Part model, mm, in its own coordinate system. A direction names the side the tool comes from. Round coordinates to 2 decimals unless told otherwise and drop trailing zeros. Write each loop counter-clockwise with the first axis right and the second up, starting at its lowest first coordinate (ties: lowest second). Pieces come first, ordered by that corner, then holes.
```python
from build123d import *

# Parameters (mm, degrees)
SKETCH1_W                = 57
SKETCH1_H                = 57
EXTRUDE1_DEPTH           = 76
F_5_0_5_DIAMETER_HOLE1_D = 5
SKETCH6_R                = 4
SKETCH6_R_2              = 2.5
EXTRUDE4_DEPTH           = 71
FILLET1_R                = 5
SKETCH7_R                = 3
EXTRUDE5_DEPTH           = 101
SKETCH8_R                = 19.05
EXTRUDE6_DEPTH           = 3
FILLET2_R                = 1
SKETCH9_R                = 5.5
BOSS_EXTRUDE1_DEPTH      = 388
CHAMFER1_SIZE            = 0.5
SKETCH10_R               = 4
BOSS_EXTRUDE2_DEPTH      = 10
CHAMFER2_SIZE            = 0.5


with BuildPart() as part:
    # Sketch1 → Extrude1 (new body)
    with BuildSketch(Plane(origin=(0, 0, 0), x_dir=(1, 0, 0), z_dir=(0, 1, 0))):
        Rectangle(SKETCH1_W, SKETCH1_H)
    extrude(amount=EXTRUDE1_DEPTH)

    # Ø5.0 (5) Diameter Hole1 (through all)
    with Locations(Plane.XZ):
        with Locations((-23.5, 23.5), (23.5, 23.5), (23.5, -23.5), (-23.5, -23.5)):
            Hole(F_5_0_5_DIAMETER_HOLE1_D / 2)

    # Sketch6 → Extrude4 (cut)
    # profile 1 of 12: a face of its own
    with BuildSketch(Plane(origin=(0, 76, 0), x_dir=(1, 0, 0), z_dir=(0, 1, 0))):
        Polygon((-28.5, 28.5), (-19.5, 28.5), (-19.5, 32.511741208), (-33.908905561, 32.511741208), (-33.908905561, 19.5), (-28.5, 19.5), align=None)
    # profile 2 of 12: a face of its own
    with BuildSketch(Plane(origin=(0, 76, 0), x_dir=(1, 0, 0), z_dir=(0, 1, 0))):
        with BuildLine():
            ThreePointArc((-23.5, 19.5), (-26.328427125, 26.328427125), (-19.5, 23.5))
            Line((-19.5, 23.5), (-19.5, 28.5))
            Line((-19.5, 28.5), (-28.5, 28.5))
            Line((-28.5, 28.5), (-28.5, 19.5))
            Line((-28.5, 19.5), (-23.5, 19.5))
        make_face()
    # profile 3 of 12: a face of its own
    with BuildSketch(Plane(origin=(0, 76, 0), x_dir=(1, 0, 0), z_dir=(0, 1, 0))):
        with Locations((-23.5, 23.5)):
            Circle(SKETCH6_R)
        with Locations(Location((-23.5, 23.5, 0), (0, 0, 90))):
            Circle(SKETCH6_R_2, mode=Mode.SUBTRACT)
    # profile 4 of 12: a face of its own
    with BuildSketch(Plane(origin=(0, 76, 0), x_dir=(1, 0, 0), z_dir=(0, 1, 0))):
        Polygon((19.5, 36.471560472), (19.5, 28.5), (28.5, 28.5), (28.5, 19.5), (41.168352552, 19.5), (41.168352552, 36.471560472), align=None)
    # profile 5 of 12: a face of its own
    with BuildSketch(Plane(origin=(0, 76, 0), x_dir=(1, 0, 0), z_dir=(0, 1, 0))):
        with BuildLine():
            Line((28.5, 28.5), (19.5, 28.5))
            Line((19.5, 28.5), (19.5, 23.5))
            ThreePointArc((19.5, 23.5), (23.5, 27.5), (27.5, 23.5))
            ThreePointArc((27.5, 23.5), (26.328427125, 20.671572875), (23.5, 19.5))
            Line((23.5, 19.5), (28.5, 19.5))
            Line((28.5, 19.5), (28.5, 28.5))
        make_face()
    # profile 6 of 12: a face of its own
    with BuildSketch(Plane(origin=(0, 76, 0), x_dir=(1, 0, 0), z_dir=(0, 1, 0))):
        with Locations((23.5, 23.5)):
            Circle(SKETCH6_R)
        with Locations(Location((23.5, 23.5, 0), (0, 0, 90))):
            Circle(SKETCH6_R_2, mode=Mode.SUBTRACT)
    # profile 7 of 12: a face of its own
    with BuildSketch(Plane(origin=(0, 76, 0), x_dir=(1, 0, 0), z_dir=(0, 1, 0))):
        with Locations((23.5, -23.5)):
            Circle(SKETCH6_R)
        with Locations(Location((23.5, -23.5, 0), (0, 0, 90))):
            Circle(SKETCH6_R_2, mode=Mode.SUBTRACT)
    # profile 8 of 12: a face of its own
    with BuildSketch(Plane(origin=(0, 76, 0), x_dir=(1, 0, 0), z_dir=(0, 1, 0))):
        with BuildLine():
            Line((28.5, -28.5), (28.5, -19.5))
            Line((28.5, -19.5), (23.5, -19.5))
            ThreePointArc((23.5, -19.5), (26.328427125, -20.671572875), (27.5, -23.5))
            ThreePointArc((27.5, -23.5), (23.5, -27.5), (19.5, -23.5))
            Line((19.5, -23.5), (19.5, -28.5))
            Line((19.5, -28.5), (28.5, -28.5))
        make_face()
    # profile 9 of 12: a face of its own
    with BuildSketch(Plane(origin=(0, 76, 0), x_dir=(1, 0, 0), z_dir=(0, 1, 0))):
        Polygon((44.252209519, -19.5), (28.5, -19.5), (28.5, -28.5), (19.5, -28.5), (19.5, -40.050429997), (44.252209519, -40.050429997), align=None)
    # profile 10 of 12: a face of its own
    with BuildSketch(Plane(origin=(0, 76, 0), x_dir=(1, 0, 0), z_dir=(0, 1, 0))):
        Polygon((-28.5, -28.5), (-28.5, -19.5), (-37.670786859, -19.5), (-37.670786859, -37.828231874), (-19.5, -37.828231874), (-19.5, -28.5), align=None)
    # profile 11 of 12: a face of its own
    with BuildSketch(Plane(origin=(0, 76, 0), x_dir=(1, 0, 0), z_dir=(0, 1, 0))):
        with BuildLine():
            Line((-23.5, -19.5), (-28.5, -19.5))
            Line((-28.5, -19.5), (-28.5, -28.5))
            Line((-28.5, -28.5), (-19.5, -28.5))
            Line((-19.5, -28.5), (-19.5, -23.5))
            ThreePointArc((-19.5, -23.5), (-26.328427125, -26.328427125), (-23.5, -19.5))
        make_face()
    # profile 12 of 12: a face of its own
    with BuildSketch(Plane(origin=(0, 76, 0), x_dir=(1, 0, 0), z_dir=(0, 1, 0))):
        with Locations((-23.5, -23.5)):
            Circle(SKETCH6_R)
        with Locations(Location((-23.5, -23.5, 0), (0, 0, 90))):
            Circle(SKETCH6_R_2, mode=Mode.SUBTRACT)
    extrude(amount=-EXTRUDE4_DEPTH, mode=Mode.SUBTRACT)

    # Fillet1
    fillet1_edges = [part.edges().sort_by_distance(p)[0] for p in [
        (-28.5, 2.5, 28.5),
        (-28.5, 2.5, -28.5),
        (28.5, 2.5, -28.5),
        (28.5, 2.5, 28.5),
    ]]
    fillet(fillet1_edges, radius=FILLET1_R)



with BuildPart() as body_2:
    # Sketch7 → Extrude5 (new body)
    with BuildSketch(Plane(origin=(0, 76, 0), x_dir=(1, 0, 0), z_dir=(0, 1, 0))):
        with Locations(Location((0, 0, 0), (0, 0, 270))):
            Circle(SKETCH7_R)
    extrude(amount=-EXTRUDE5_DEPTH)


with BuildPart() as part_1:
    add(part.part)

    add(body_2.part)  # Extrude6 merges body 2
    # Sketch8 → Extrude6 (add)
    with BuildSketch(Plane.XZ):
        with Locations(Location((0, 0, 0), (0, 0, 270))):
            Circle(SKETCH8_R)
    extrude(amount=EXTRUDE6_DEPTH)

    # Fillet2
    fillet2_edges = [part_1.edges().sort_by_distance(p)[0] for p in [
        (-28.5, 40.5, 19.5),
        (0, 76, 28.5),
        (-19.5, 40.5, 28.5),
        (-19.5, 76, 26),
        (-20.671572875, 76, 20.671572875),
        (-26, 76, 19.5),
        (-28.5, 76, 0),
        (-28.5, 40.5, -19.5),
        (-19.5, 40.5, -28.5),
        (-19.5, 76, -26),
        (-26, 76, -19.5),
        (-20.671572875, 76, -20.671572875),
        (0, 76, -28.5),
        (19.5, 76, -26),
        (26, 76, -19.5),
        (20.671572875, 76, -20.671572875),
        (19.5, 40.5, -28.5),
        (28.5, 40.5, -19.5),
        (19.5, 40.5, 28.5),
        (28.5, 76, 0),
        (26, 76, 19.5),
        (19.5, 76, 26),
        (20.671572875, 76, 20.671572875),
        (28.5, 40.5, 19.5),
    ]]
    fillet(fillet2_edges, radius=FILLET2_R)

    # Sketch9 → Boss-Extrude1 (add)
    with BuildSketch(Plane.XZ):
        with Locations(Location((0, 0, 0), (0, 0, 90))):
            Circle(SKETCH9_R)
    extrude(amount=BOSS_EXTRUDE1_DEPTH)

    # Chamfer1
    chamfer1_edges = [part_1.edges().sort_by_distance(p)[0] for p in [
        (0, -388, -5.5),
    ]]
    chamfer(chamfer1_edges, length=CHAMFER1_SIZE)

    # Sketch10 → Boss-Extrude2 (add)
    with BuildSketch(Plane.XZ.offset(388)):
        with Locations(Location((0, 0, 0), (0, 0, 270))):
            Circle(SKETCH10_R)
    extrude(amount=BOSS_EXTRUDE2_DEPTH)

    # Chamfer2
    chamfer2_edges = [part_1.edges().sort_by_distance(p)[0] for p in [
        (0, -398, 4),
    ]]
    chamfer(chamfer2_edges, length=CHAMFER2_SIZE)


solid = part_1.part
```
Q1. Cut at A-A on y = 37.5. Write the cut outline in (x, z), plus the area to 3 significant figures.
Values follow:
outline: (-28.5, -18.5) arc R1 ccw to (-27.5, -19.5) - (-23.5, -19.5) arc R4 cw to (-19.5, -23.5) - (-19.5, -27.5) arc R1 ccw to (-18.5, -28.5) - (18.5, -28.5) arc R1 ccw to (19.5, -27.5) - (19.5, -23.5) arc R4 cw to (23.5, -19.5) - (27.5, -19.5) arc R1 ccw to (28.5, -18.5) - (28.5, 18.5) arc R1 ccw to (27.5, 19.5) - (23.5, 19.5) arc R4 cw to (19.5, 23.5) - (19.5, 27.5) arc R1 ccw to (18.5, 28.5) - (-18.5, 28.5) arc R1 ccw to (-19.5, 27.5) - (-19.5, 23.5) arc R4 cw to (-23.5, 19.5) - (-27.5, 19.5) arc R1 ccw to (-28.5, 18.5) - close
area: 2,940 mm2
Q2. Wall check: L1, parallel to Z at x = -23.5, y = 3.3; L2, parallel to Z at x = -23, y = 3. Give the ranges that are in metal, low to high.
Values follow:
L1: z = -28.5 to -26, -21 to 21, 26 to 28.5
L2: z = -28.5 to -25.95, -21.05 to 21.05, 25.95 to 28.5
Q3. Which spindle directions (+Z, -Z, +X, -X, +Y, -Y) get a long thin tool onto all of the face, cutting with end or side? Do faces 1 (the cylindrical face through (5.37, -192.56, -1.19)), 2 (the flat face through (26, 5, 26)), 3 (the flat face through (-26, 5, 25)). Say none if no direction does.
Values follow:
face 1: -Y
face 2: +Z, +X, +Y
face 3: +Z, -X, +Y
Q4. Cut at C-C on y = -46. Write the cut outline in (x, z).
Values follow:
outline: circle Ø11 at (0, 0)
Q5. Drop flat-ended pins along their axis: pin 1 (3 mm diameter, centred on x = 25, y = 32.5, fed in from +Z); pin 2 (1.2 mm diameter, centred on x = -26, y = 37.5, fed in from -Z); pin 3 (5 mm diameter, centred on x = -25, z = 23, fed in from +Y); pin 4 (4.5 mm diameter, centred on x = -23.5, z = -23.5, fed in from -Y). Give the stop position or say it passes through.
Values follow:
pin 1: stops at z = 19.5
pin 2: stops at z = -19.5
pin 3: stops at y = 5
pin 4: passes through
Q6. Cut at B-B on z = 9.5. Write the cut outline in (x, y).
Values follow:
outline: (-28.5, 0) - (-16.51, 0) - (-16.51, -3) - (16.51, -3) - (16.51, 0) - (28.5, 0) - (28.5, 75) arc R1 ccw to (27.5, 76) - (-27.5, 76) arc R1 ccw to (-28.5, 75) - close
